```python
from build123d import *

# Parameters (mm, degrees)
F0_R     = 57
F1_DEPTH = 10
F2_R     = 55
F3_DEPTH = 25
F4_R     = 2.5
F4_R_2   = 1.5
F5_DEPTH = 10
F6_R     = 5
F7_R     = 5


with BuildPart() as f1:
    # F0 (on Top) → F1 (new body)
    with BuildSketch(Plane.XY):
        Circle(F0_R)
    extrude(amount=F1_DEPTH)

    # F2 (on Top) → F3 (cut)
    with BuildSketch(Plane.XY):
        Circle(F2_R)
    extrude(amount=F3_DEPTH, mode=Mode.SUBTRACT)

    # F4 (on Top) → F5 (join)
    with BuildSketch(Plane.XY):
        with Locations((58.5, 0)):
            Circle(F4_R)
        with Locations((58.5, 0)):
            Circle(F4_R_2, mode=Mode.SUBTRACT)
        with Locations((-58.5, 0)):
            Circle(F4_R)
        with Locations((-58.5, 0)):
            Circle(F4_R_2, mode=Mode.SUBTRACT)
    extrude(amount=F5_DEPTH)

    # F6
    f6_edges = [f1.edges().sort_by_distance(p)[0] for p in [
        (-56.965812, -1.973896, 5),
        (-56.965812, 1.973896, 5),
    ]]
    fillet(f6_edges, radius=F6_R)

    # F7
    f7_edges = [f1.edges().sort_by_distance(p)[0] for p in [
        (56.965812, -1.973896, 5),
        (56.965812, 1.973896, 5),
    ]]
    fillet(f7_edges, radius=F7_R)


solid = f1.part
```
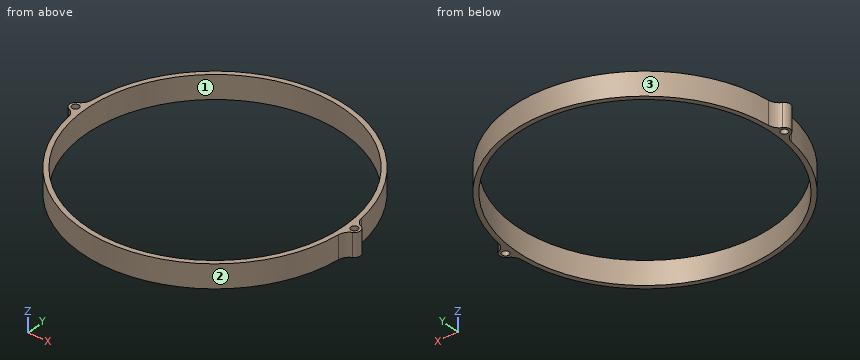
Input: part model. Units: mm. Frame: model coordinates. Face numbers are marked on the shaded views. Round coordinates to 2 decimals unless told otherwise and drop trailing zeros. Loops run counter-clockwise (first coordinate to the right, second up) from the corner with the lowest first, then second, coordinate; pieces in that order, holes last.
1) Section query B-B on y = 40.5. Return the cut outline in (x, z), plus the area to 3 significant figures.
Ans:
outline: (-40.11, 0) - (-37.21, 0) - (-37.21, 10) - (-40.11, 10) - close; (37.21, 0) - (40.11, 0) - (40.11, 10) - (37.21, 10) - close
area: 57.9 mm2
2) Section query A-A on x = 0. Return the cut outline in (y, z).
Ans:
outline: (-57, 0) - (-55, 0) - (-55, 10) - (-57, 10) - close; (55, 0) - (57, 0) - (57, 10) - (55, 10) - close
3) Pull-direction query (Y, two-part tool) for the marked faces 1, 2 and 3; classes: released by +Y, released by -Y, zero draft, split by the parting line, or undercut.
Ans:
face 1: undercut
face 2: released by -Y
face 3: released by +Y
4) Pin query (flat end, axial travel): pin 1 (6 mm diameter, centred on x = 28.5, z = 2, fed in from -Y); pin 2 (1.5 mm diameter, centred on x = -17, z = 5.5, fed in from +Y); pin 3 (5 mm diameter, centred on x = -58.5, y = 0, fed in from +Z). Return the tip coordinate at first contact, or that it passes through.
Ans:
pin 1: stops at y = -50.98
pin 2: stops at y = 54.63
pin 3: stops at z = 10
5) Material intervals for line 1 (Y direction, x = 1, z = 9.25); line 2 (Y direction, x = -31, z = 4); line 3 (X direction, y = -3, z = 1.25), sorted ascending.
Ans:
line 1: y = -56.99 to -54.99, 54.99 to 56.99
line 2: y = -47.83 to -45.43, 45.43 to 47.83
line 3: x = -58.4 to -54.92, 54.92 to 58.4
6) Section query C-C on y = 0. Return the cut outline in (x, z), plus the area to 3 significant figures.
Ans:
outline: (-61, 0) - (-60, 0) - (-60, 10) - (-61, 10) - close; (-57, 0) - (-55, 0) - (-55, 10) - (-57, 10) - close; (55, 0) - (57, 0) - (57, 10) - (55, 10) - close; (60, 0) - (61, 0) - (61, 10) - (60, 10) - close
area: 60.0 mm2
7) Section query D-D on z = 5.5. Count the separate pieces of the cut face and the enclosed holes in it, plus the area to 3 significant figures.
Ans:
separate pieces: 1
enclosed holes: 3
area: 734 mm2
